Build history of the part. All positions in model axes, mm. Round coordinates to 2 decimals unless told otherwise and drop trailing zeros. Write each loop counter-clockwise with the first axis right and the second up, starting at its lowest first coordinate (ties: lowest second). Pieces come first, ordered by that corner, then holes. Notation, with made-up numbers: (8, -15) -> (40, -15) arc R31 cw to (40, 16) -> close; hole circle Ø11 at (54.25, -23). An arc over 180 degrees is marked (long way). Answer in a Markdown table with one row per item.
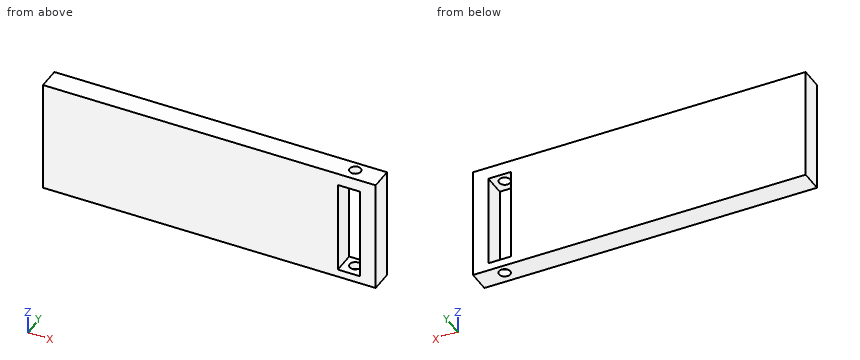
```python
from build123d import *

# Parameters (mm, degrees)
SKETCH1_W           = 150
SKETCH1_H           = 51
BOSS_EXTRUDE1_DEPTH = 10
SKETCH2_W           = 10.1
SKETCH2_H           = 42
CUT_EXTRUDE1_DEPTH  = 80.845162659
SKETCH5_R           = 2.5
CUT_EXTRUDE4_DEPTH  = 92.246917756


with BuildPart() as part:
    # Sketch1 → Boss-Extrude1 (new body)
    with BuildSketch(Plane(origin=(0, 0, 0), x_dir=(1, 0, 0), z_dir=(0, 1, 0))):
        Rectangle(SKETCH1_W, SKETCH1_H)
    extrude(amount=BOSS_EXTRUDE1_DEPTH)

    # Sketch2 → Cut-Extrude1 (cut, through all)
    with BuildSketch(Plane(origin=(0, 10, 0), x_dir=(1, 0, 0), z_dir=(0, 1, 0))):
        with Locations((63, 1)):
            Rectangle(SKETCH2_W, SKETCH2_H)
    extrude(amount=-CUT_EXTRUDE1_DEPTH, mode=Mode.SUBTRACT)

    # Sketch5 → Cut-Extrude4 (cut, through all)
    with BuildSketch(Plane.XY.offset(25.5)):
        with Locations((63, 5.515561539)):
            Circle(SKETCH5_R)
    extrude(amount=-CUT_EXTRUDE4_DEPTH, mode=Mode.SUBTRACT)


solid = part.part
```
Q1. Drop a flat-ended pin along its axis: P1, Ø4.5, axis at x = 63, y = 5.52, coming from the -Z side. Give the stop position or say it passes through.
A:
| item | result |
|---|---|
| P1 | through |
Q2. Wall check: line 1 (X direction, y = 8.5, z = -11.5); line 2 (Y direction, x = 63, z = -23); line 3 (Z direction, x = 60.5, y = 0.5). Give the ranges that are in metal, low to high. Write a range as [from, to].
A:
| item | result |
|---|---|
| line 1 | [-75, 57.95], [68.05, 75] |
| line 2 | [0, 3.02], [8.02, 10] |
| line 3 | [-25.5, -22], [20, 25.5] |
Q3. Saw through at A-A on x = 63. Write the cut outline in (y, z).
A:
| item | result |
|---|---|
| outline | (0, -25.5) -> (3.02, -25.5) -> (3.02, -22) -> (0, -22) -> close; (0, 20) -> (3.02, 20) -> (3.02, 25.5) -> (0, 25.5) -> close; (8.02, -25.5) -> (10, -25.5) -> (10, -22) -> (8.02, -22) -> close; (8.02, 20) -> (10, 20) -> (10, 25.5) -> (8.02, 25.5) -> close |
Q4. Saw through at B-B on z = 13. Write the cut outline in (x, y).
A:
| item | result |
|---|---|
| outline | (-75, 0) -> (57.95, 0) -> (57.95, 10) -> (-75, 10) -> close; (68.05, 0) -> (75, 0) -> (75, 10) -> (68.05, 10) -> close |
